Can you work these out from the model? Positions are in its coordinate system, mm. Round coordinates to 2 decimals unless told otherwise and drop trailing zeros. Loops run counter-clockwise (first coordinate to the right, second up) from the corner with the lowest first, then second, coordinate; pieces in that order, holes last. Notation, with made-up numbers: (56.25, -10.5) -> (90.25, -10.5) arc R14 ccw to (90.25, -3.5) -> close; hole circle Ø7 at (25.5, 6.25). An arc over 180 degrees is marked (long way). Write each question's results on one line, items separated by ' | '.
from build123d import *

# Parameters (mm, degrees)
SKETCH1_W           = 114.3
SKETCH1_H           = 190.5
SKETCH1_W_2         = 88.9
SKETCH1_H_2         = 139.7
BOSS_EXTRUDE1_DEPTH = 3.175
SKETCH2_R           = 2.54
CUT_EXTRUDE1_DEPTH  = 4.7625
FILLET1_R           = 2.54
FILLET2_R           = 2.54


with BuildPart() as part:
    # Sketch1 → Boss-Extrude1 (new body)
    with BuildSketch(Plane(origin=(0, 0, 0), x_dir=(1, 0, 0), z_dir=(0, 1, 0))):
        Rectangle(SKETCH1_W, SKETCH1_H)
        Rectangle(SKETCH1_W_2, SKETCH1_H_2, mode=Mode.SUBTRACT)
    extrude(amount=BOSS_EXTRUDE1_DEPTH)

    # Sketch2 → Cut-Extrude1 (cut)
    with BuildSketch(Plane(origin=(0, 3.175, 0), x_dir=(1, 0, 0), z_dir=(0, 1, 0))):
        with Locations(Location((19.05, -82.55, 0), (0, 0, 270))):
            Circle(SKETCH2_R)
        with Locations(Location((19.05, 82.55, 0), (0, 0, 270))):
            Circle(SKETCH2_R)
        with Locations(Location((-19.05, -82.55, 0), (0, 0, 270))):
            Circle(SKETCH2_R)
        with Locations(Location((-19.05, 82.55, 0), (0, 0, 270))):
            Circle(SKETCH2_R)
    extrude(amount=-CUT_EXTRUDE1_DEPTH, mode=Mode.SUBTRACT)

    # Fillet1
    fillet1_edges = [part.edges().sort_by_distance(p)[0] for p in [
        (-44.45, 1.5875, -69.85),
        (-44.45, 1.5875, 69.85),
        (44.45, 1.5875, 69.85),
        (44.45, 1.5875, -69.85),
    ]]
    fillet(fillet1_edges, radius=FILLET1_R)

    # Fillet2
    fillet2_edges = [part.edges().sort_by_distance(p)[0] for p in [
        (-57.15, 1.5875, -95.25),
        (57.15, 1.5875, -95.25),
        (57.15, 1.5875, 95.25),
        (-57.15, 1.5875, 95.25),
    ]]
    fillet(fillet2_edges, radius=FILLET2_R)


solid = part.part
1. Will these pins go through, and if not, where does the flat tip stop? pin 1 (6 mm diameter, centred on x = 19.05, z = -82.55, fed in from -Y); pin 2 (12 mm diameter, centred on x = 37.5, z = -59, fed in from +Y).
Final values:
pin 1: y = 0 | pin 2: through
2. We'd pull the mould along Z, two halves only. Please class faces 1 (the face through (-18.938, 1.61, -85.088)), 2 (the face through (-52, 0, -1)): pulls with the +Z half, pulls with the -Z half, needs draft (parallel to the pull), parting line crosses it, or undercut.
Final values:
face 1: undercut | face 2: needs draft
3. If we section it at B-B (x = 38): List the corners of the cut face in (y, z) for me (3 decimals), then the cut area to 3 significant figures.
Final values:
outline: (0, -95.25) -> (3.175, -95.25) -> (3.175, -69.85) -> (0, -69.85) -> close; (0, 69.85) -> (3.175, 69.85) -> (3.175, 95.25) -> (0, 95.25) -> close | area: 161 mm2
4. If we section it at D-D (x = 19.05): List the corners of the cut face in (y, z) for me (3 decimals).
Final values:
outline: (0, -95.25) -> (3.175, -95.25) -> (3.175, -85.09) -> (0, -85.09) -> close; (0, -80.01) -> (3.175, -80.01) -> (3.175, -69.85) -> (0, -69.85) -> close; (0, 69.85) -> (3.175, 69.85) -> (3.175, 80.01) -> (0, 80.01) -> close; (0, 85.09) -> (3.175, 85.09) -> (3.175, 95.25) -> (0, 95.25) -> close
5. If we section it at A-A (z = -82.55): List the corners of the cut face in (x, y) for me (3 decimals).
Final values:
outline: (-57.15, 0) -> (-21.59, 0) -> (-21.59, 3.175) -> (-57.15, 3.175) -> close; (-16.51, 0) -> (16.51, 0) -> (16.51, 3.175) -> (-16.51, 3.175) -> close; (21.59, 0) -> (57.15, 0) -> (57.15, 3.175) -> (21.59, 3.175) -> close
6. If we section it at C-C (y = 1.2): List the corners of the cut face in (x, z) for me, then the cut area to 3 significant figures.
Final values:
outline: (-57.15, -92.71) arc R2.54 ccw to (-54.61, -95.25) -> (54.61, -95.25) arc R2.54 ccw to (57.15, -92.71) -> (57.15, 92.71) arc R2.54 ccw to (54.61, 95.25) -> (-54.61, 95.25) arc R2.54 ccw to (-57.15, 92.71) -> close; hole (-44.45, -67.31) arc R2.54 ccw to (-41.91, -69.85) -> (41.91, -69.85) arc R2.54 ccw to (44.45, -67.31) -> (44.45, 67.31) arc R2.54 ccw to (41.91, 69.85) -> (-41.91, 69.85) arc R2.54 ccw to (-44.45, 67.31) -> close; hole circle Ø5.08 at (-19.05, -82.55); hole circle Ø5.08 at (-19.05, 82.55); hole circle Ø5.08 at (19.05, -82.55); hole circle Ø5.08 at (19.05, 82.55) | area: 9,270 mm2
7. Please list where these lines run through material, in increasing order: line 1 (X direction, y = 2.45, z = -82.55); line 2 (X direction, y = 1.9, z = 55.5); line 3 (Z direction, x = -2, y = 2.5). Write a range as from..to.
Final values:
line 1: -57.15..-21.59, -16.51..16.51, 21.59..57.15 | line 2: -57.15..-44.45, 44.45..57.15 | line 3: -95.25..-69.85, 69.85..95.25
